Read the model definition and answer for the solid it produces. Units are mm, in the model's axes. A direction names the side the tool comes from. Round coordinates to 2 decimals unless told otherwise and drop trailing zeros. Write each loop counter-clockwise with the first axis right and the second up, starting at its lowest first coordinate (ties: lowest second). Pieces come first, ordered by that corner, then holes. Notation, with made-up numbers: (8.25, -3.5) -> (67.25, -3.5) arc R33 ccw to (67.25, 25.5) -> close; hole circle Ø11 at (-14, 83.5). An arc over 180 degrees is marked (long way). Return JSON: item names as keys, results as strings.
from build123d import *

# Parameters (mm, degrees)
F0_W     = 24
F0_H     = 11
F1_DEPTH = 5
F2_R     = 0.75
F3_DEPTH = 1
F5_DEPTH = 11.001


with BuildPart() as f1:
    # F0 (on Top) → F1 (new body)
    with BuildSketch(Plane.XY):
        Rectangle(F0_W, F0_H)
    extrude(amount=F1_DEPTH)

    # F2 (on face) → F3 (cut)
    with BuildSketch(Plane.XY.offset(5)):
        with Locations((-7, -0.5)):
            Circle(F2_R)
        with Locations((7, -0.5)):
            Circle(F2_R)
    extrude(amount=-F3_DEPTH, mode=Mode.SUBTRACT)

    # F4 (on face) → F5 (cut, through all)
    with BuildSketch(Plane.XZ.offset(5.5)):
        Polygon((-12, 0), (9.848078, 0), (-9.848078, 3.472964), (-12, 3.472964), align=None)
    extrude(amount=-F5_DEPTH, mode=Mode.SUBTRACT)


solid = f1.part
Item 1: Section B-B (x = 7) is taken. Give the vertices of the cut face in (y, z).
Worked answers:
{"outline": "(-5.5, 0.5) -> (5.5, 0.5) -> (5.5, 5) -> (0.25, 5) -> (0.25, 4) -> (-1.25, 4) -> (-1.25, 5) -> (-5.5, 5) -> close"}
Item 2: A tool of negligible diameter and unlimited length cuts with its end or side. For faces 4 (the flat face through (7, 0, 4)), 5 (the flat face through (11, 0, 0)), from which of +Z, -Z, +X, -X, +Y, -Y can it reach the whole face along a straight path? Write none if from no direction.
Worked answers:
{"face 4": "+Z", "face 5": "-Z, +X, -X, +Y, -Y"}
Item 3: Section A-A (y = -0.5) is taken. Give the vertices of the cut face in (x, z), then the cut area to 3 significant figures.
Worked answers:
{"outline": "(-12, 3.47) -> (-9.85, 3.47) -> (9.85, 0) -> (12, 0) -> (12, 5) -> (7.75, 5) -> (7.75, 4) -> (6.25, 4) -> (6.25, 5) -> (-6.25, 5) -> (-6.25, 4) -> (-7.75, 4) -> (-7.75, 5) -> (-12, 5) -> close", "area": "75.3 mm2"}
Item 4: Section D-D (z = 0.7) is taken. Give the vertices of the cut face in (x, y), then the cut area to 3 significant figures.
Worked answers:
{"outline": "(5.88, -5.5) -> (12, -5.5) -> (12, 5.5) -> (5.88, 5.5) -> close", "area": "67.3 mm2"}
Item 5: Section C-C (y = 1) is taken. Give the vertices of the cut face in (x, z), then the cut area to 3 significant figures.
Worked answers:
{"outline": "(-12, 3.47) -> (-9.85, 3.47) -> (9.85, 0) -> (12, 0) -> (12, 5) -> (-12, 5) -> close", "area": "78.3 mm2"}
Item 6: For a pull along Y with two mould halves and no side action, classify faces 1 (the cylindrical face through (-7.75, -0.47, 4.51)), 2 (the flat face through (2, 5.5, 3)), 3 (the flat face through (-11, 0, 3.473)) as released by +Y, released by -Y, zero draft, split by the parting line, or undercut.
Worked answers:
{"face 1": "undercut", "face 2": "released by +Y", "face 3": "zero draft"}
Item 7: Flat-ended cylindrical pins translate along their axes: pin 1 (1.6 mm diameter, centred on x = 7, y = -0.5, fed in from +Z); pin 2 (3 mm diameter, centred on x = 4.5, y = 0.5, fed in from -Z); pin 3 (1.1 mm diameter, centred on x = -11, y = 0.5, fed in from -Z); pin 4 (1.7 mm diameter, centred on x = -7, y = -0.5, fed in from -Z). Find the tip coordinate at first contact, or state that the pin passes through.
Worked answers:
{"pin 1": "stops at z = 5", "pin 2": "stops at z = 0.68", "pin 3": "stops at z = 3.47", "pin 4": "stops at z = 2.82"}
Item 8: Straight lines are drawn through the part: L1, parallel to Y at x = -7, z = 4.7; L2, parallel to Z at x = 5.5, y = -4.25; L3, parallel to Z at x = -7.5, y = 0.75. For each, find the intervals that lie inside material, in ascending order. Write a range as [from, to].
Worked answers:
{"L1": "y = [-5.5, -1.25], [0.25, 5.5]", "L2": "z = [0.77, 5]", "L3": "z = [3.06, 5]"}
